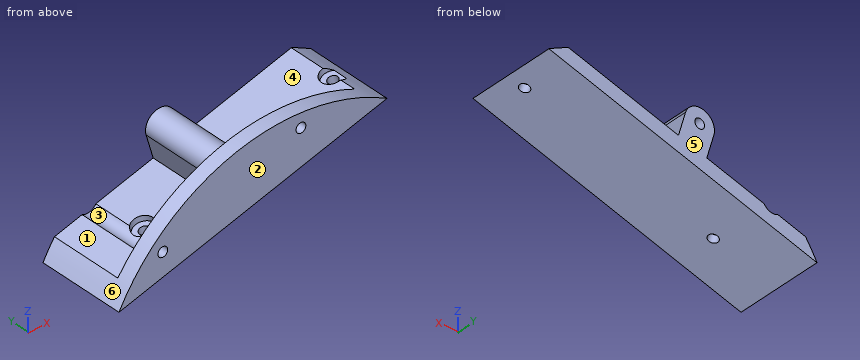
from build123d import *

# Parameters (mm, degrees)
SKETCH1_R           = 1.65
BOSS_EXTRUDE1_DEPTH = 5
BOSS_EXTRUDE2_DEPTH = 25
SKETCH3_R           = 1.65
CUT_EXTRUDE1_DEPTH  = 31.640005718
SKETCH4_R           = 3.5
CUT_EXTRUDE2_DEPTH  = 2
SKETCH5_R           = 67.5
SKETCH5_R_2         = 66.25
CUT_EXTRUDE3_DEPTH  = 31.0000001
SKETCH6_R           = 1.65
BOSS_EXTRUDE3_DEPTH = 30
CUT_EXTRUDE4_START  = -3
CUT_EXTRUDE4_DEPTH  = 2.6


with BuildPart() as part:
    # Sketch1 → Boss-Extrude1 (new body)
    with BuildSketch(Plane(origin=(0, 0, 0), x_dir=(1, 0, 0), z_dir=(0, 1, 0))):
        with BuildLine():
            ThreePointArc((-58.769725256, -31.225340563), (-18.644922026, -63.884813396), (32.748082014, -57.935012077))
            Line((32.748082014, -57.935012077), (-58.769725256, -31.225340563))
        make_face()
        with Locations((-43.522422382, -43.522422382)):
            Circle(SKETCH1_R, mode=Mode.SUBTRACT)
        with Locations((3.221278107, -61.465647864)):
            Circle(SKETCH1_R, mode=Mode.SUBTRACT)
    extrude(amount=BOSS_EXTRUDE1_DEPTH)

    # Sketch2 → Boss-Extrude2 (add)
    with BuildSketch(Plane(origin=(0, 5, 0), x_dir=(1, 0, 0), z_dir=(0, 1, 0))):
        with BuildLine():
            Line((-58.769725256, -31.225340563), (32.748082014, -57.935012077))
            ThreePointArc((32.748082014, -57.935012077), (29.480015366, -59.664320946), (26.120952253, -61.20946294))
            Line((26.120952253, -61.20946294), (-40.494047404, -41.767730103))
            ThreePointArc((-40.494047404, -41.767730103), (-42.54184797, -40.162589972), (-45.131562946, -40.414261085))
            Line((-45.131562946, -40.414261085), (-54.944236671, -37.550410872))
            ThreePointArc((-54.944236671, -37.550410872), (-56.94486731, -34.441030575), (-58.769725256, -31.225340563))
        make_face()
    extrude(amount=BOSS_EXTRUDE2_DEPTH)

    # Sketch3 → Cut-Extrude1 (cut, through all)
    with BuildSketch(Plane(origin=(-14.411642209, 0, 49.379936906), x_dir=(0.959952117, 0, 0.280164118), z_dir=(-0.280164118, 0, 0.959952117))):
        with Locations((41.56355859, 14)):
            Circle(SKETCH3_R)
        with Locations((-24.93644141, 14)):
            Circle(SKETCH3_R)
    extrude(amount=-CUT_EXTRUDE1_DEPTH, mode=Mode.SUBTRACT)

    # Sketch4 → Cut-Extrude2 (cut)
    with BuildSketch(Plane(origin=(-14.411642209, 0, 49.379936906), x_dir=(0.959952117, 0, 0.280164118), z_dir=(-0.280164118, 0, 0.959952117))):
        with Locations((41.56355859, 14)):
            Circle(SKETCH4_R)
        with Locations((-24.93644141, 14)):
            Circle(SKETCH4_R)
    extrude(amount=-CUT_EXTRUDE2_DEPTH, mode=Mode.SUBTRACT)

    # Sketch5 → Cut-Extrude3 (cut, through all)
    with BuildSketch(Plane.XZ):
        Circle(SKETCH5_R)
        Circle(SKETCH5_R_2, mode=Mode.SUBTRACT)
    extrude(amount=-CUT_EXTRUDE3_DEPTH, mode=Mode.SUBTRACT)

    # Sketch6 → Boss-Extrude3 (add)
    with BuildSketch(Plane(origin=(0, 0, 0), x_dir=(1, 0, 0), z_dir=(0, 1, 0))):
        with BuildLine():
            Line((-23.475659958, -55.618568944), (-21.086364171, -47.431904754))
            Line((-21.086364171, -47.431904754), (-11.486842999, -50.23354593))
            Line((-11.486842999, -50.23354593), (-13.876138786, -58.42021012))
            ThreePointArc((-13.876138786, -58.42021012), (-20.07671996, -61.819150118), (-23.475659958, -55.618568944))
        make_face()
        with Locations((-18.675899372, -57.019389532)):
            Circle(SKETCH6_R, mode=Mode.SUBTRACT)
    extrude(amount=BOSS_EXTRUDE3_DEPTH)

    # Sketch7 → Cut-Extrude4 (cut)
    with BuildSketch(Plane(origin=(0, 30, 0), x_dir=(1, 0, 0), z_dir=(0, 1, 0)).offset(CUT_EXTRUDE4_START)):
        Polygon((-15.535775757, -56.547206291), (-17.514760247, -54.06387109), (-20.654883862, -54.536054331), (-21.816022987, -57.491572774), (-19.837038497, -59.974907975), (-16.696914882, -59.502724734), align=None)
    extrude(amount=-CUT_EXTRUDE4_DEPTH, mode=Mode.SUBTRACT)


solid = part.part
Build history of the part. All positions in model axes, mm. Face numbers are marked on the shaded views. A direction names the side the tool comes from. Round coordinates to 2 decimals unless told otherwise and drop trailing zeros. Write each loop counter-clockwise with the first axis right and the second up, starting at its lowest first coordinate (ties: lowest second). Pieces come first, ordered by that corner, then holes. Notation, with made-up numbers: (24, 24.5) -> (29, 24.5) arc R12 cw to (29, 41.5) -> close; hole circle Ø4 at (-2, -17). An arc over 180 degrees is marked (long way). Use one line per item in the form item = value.
Q1. Band-saw the part on A-A, the plane y = 19. Write the cut outline in (x, z).
Conclusion:
outline = (-58.37, 31.34) -> (32.35, 57.82) arc R66.25 ccw to (25.67, 61.08) -> (-11.49, 50.23) -> (-13.88, 58.42) arc R5 ccw to (-23.48, 55.62) -> (-21.09, 47.43) -> (-40.49, 41.77) arc R3.5 cw to (-45.13, 40.41) -> (-54.49, 37.68) arc R66.25 ccw to start; hole circle Ø3.3 at (-18.68, 57.02)
Q2. Two-plate mould, pull along X, no slides. Class the marked faces 4, 5 and 6: released by +X, released by -X, zero draft, split by the parting line, or undercut.
Conclusion:
face_4 = undercut
face_5 = zero draft
face_6 = split by the parting line
Q3. Tool access for the marked faces 1, 2 and 3: list every direction of +Z, -Z, +X, -X, +Y, -Y with a clear straight run to the whole face (end or side of a thin tool).
Conclusion:
face_1 = +Z, -X, +Y
face_2 = +Z, -Z, +X, -X, -Y
face_3 = +Z, +Y
Q4. Band-saw the part on B-B, the plane x = -27.5. Write the cut outline in (y, z).
Conclusion:
outline = (0, 40.35) -> (30, 40.35) -> (30, 45.56) -> (5, 45.56) -> (5, 60.27) -> (0, 60.27) -> close
Q5. Drop flat-ended pins along their axis: P1, Ø4, axis at x = -8.5, z = 45, coming from the +Y side; P2, Ø12, axis at y = 17, z = 38, coming from the -X side; P3, Ø3, axis at x = -23.5, y = 25.5, coming from the +Z side; P4, Ø3, axis at x = -18.68, z = 57.02, coming from the +Y side. Give the stop position or say it passes through.
Conclusion:
P1 = 30
P2 = -58.01
P3 = 60.75
P4 = 5
Q6. Band-saw the part on C-C, the plane z = 52. Write the cut outline in (x, y), then the cut area to 3 significant figures.
Conclusion:
outline = (-41.05, 0) -> (12.41, 0) -> (12.41, 30) -> (-5.43, 30) -> (-5.43, 5) -> (-12, 5) -> (-12, 30) -> (-22.42, 30) -> (-22.42, 5) -> (-41.05, 5) -> close
area = 974 mm²
Q7. Drill centre lines: L1, parallel to Y at x = -38.5, z = 45.5; L2, parallel to Z at x = 24.5, y = 9; L3, parallel to Z at x = -8, y = 5.5. Where is each one in solid material? Low to high.
Conclusion:
L1 = 0 to 5
L2 = 55.53 to 60.74
L3 = 46.04 to 51.25
Q8. Band-saw the part on D-D, the plane x = 19. Write the cut outline in (y, z).
Conclusion:
outline = (0, 53.92) -> (30, 53.92) -> (30, 59.13) -> (5, 59.13) -> (5, 63.47) -> (0, 63.47) -> close
